CAD build for the part. Positions are in the model's coordinates, mm. Coordinates: 2 decimals unless noted, no trailing zeros. Answer in a Markdown table with one row per item. Add a question column.
Q1. Drill centre lines: line 1 along Y through (x, z) = (-9, 0.65); line 2 along X through (y, z) = (104.2, 0.55); line 3 along Y through (x, z) = (0, 0.75). Where is each one in solid material? Low to high. Write a range as from..to.
Q2. Band-saw the part on A-A (z = 1.3). State how many separate pieces and enclosed holes the cut face has, and give its area (3 significant figures).
Q3. Pin check, flat tip, straight feed: pin 1 (6 mm diameter, centred on x = -19, y = -42, fed in from -Z). Stop position of the tip, or through.
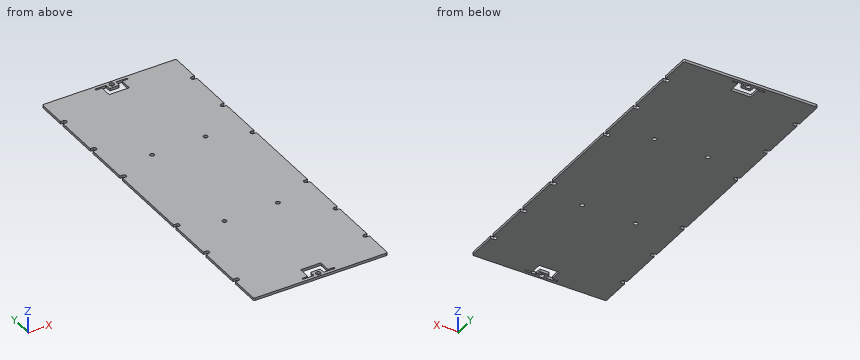
```python
from build123d import *

# Parameters (mm, degrees)
SKETCH1_W                  = 82.8
SKETCH1_H                  = 213.8
SKETCH1_R                  = 0.8
PCB_EXTRUDE_DEPTH          = 1.6
SKETCH7_W                  = 82.5
SKETCH7_H                  = 213.5
OFFSET_EDGES_DEPTH         = 1.6
CORNER_FILLETS_ON_PCB_R    = 1
SKETCH3_R                  = 1.5
SOLAR_HOLE_DEPTH           = 1.6
FILLETS_FOR_SOLAR_HOLE_R   = 0.5
M2_CLEARANCE_HOLE1_D       = 2.6
SKETCH6_W                  = 1.75
SKETCH6_H                  = 2.6
SLOTS_FOR_EDGE_HOLES_DEPTH = 1.6


with BuildPart() as part:
    # Sketch1 → pcb extrude (new body)
    with BuildSketch(Plane.XY):
        Rectangle(SKETCH1_W, SKETCH1_H)
        with Locations((-39.5, -27)):
            Circle(SKETCH1_R, mode=Mode.SUBTRACT)
        with Locations((39.5, -27)):
            Circle(SKETCH1_R, mode=Mode.SUBTRACT)
        with Locations((-39.5, 87)):
            Circle(SKETCH1_R, mode=Mode.SUBTRACT)
        with Locations((-39.5, 57)):
            Circle(SKETCH1_R, mode=Mode.SUBTRACT)
        with Locations((-39.5, 27)):
            Circle(SKETCH1_R, mode=Mode.SUBTRACT)
        with Locations((-16.5, 36.5)):
            Circle(SKETCH1_R, mode=Mode.SUBTRACT)
        with Locations((-16.5, -36.5)):
            Circle(SKETCH1_R, mode=Mode.SUBTRACT)
        with Locations((-39.5, -57)):
            Circle(SKETCH1_R, mode=Mode.SUBTRACT)
        with Locations((-39.5, -87)):
            Circle(SKETCH1_R, mode=Mode.SUBTRACT)
        with Locations((0, -104.2)):
            Circle(SKETCH1_R, mode=Mode.SUBTRACT)
        with Locations((39.5, -87)):
            Circle(SKETCH1_R, mode=Mode.SUBTRACT)
        with Locations((39.5, -57)):
            Circle(SKETCH1_R, mode=Mode.SUBTRACT)
        with Locations((16.5, -36.5)):
            Circle(SKETCH1_R, mode=Mode.SUBTRACT)
        with Locations((39.5, 27)):
            Circle(SKETCH1_R, mode=Mode.SUBTRACT)
        with Locations((16.5, 36.5)):
            Circle(SKETCH1_R, mode=Mode.SUBTRACT)
        with Locations((39.5, 57)):
            Circle(SKETCH1_R, mode=Mode.SUBTRACT)
        with Locations((39.5, 87)):
            Circle(SKETCH1_R, mode=Mode.SUBTRACT)
        with Locations((0, 104.2)):
            Circle(SKETCH1_R, mode=Mode.SUBTRACT)
    extrude(amount=PCB_EXTRUDE_DEPTH)

    # Sketch7 → Offset Edges (cut)
    with BuildSketch(Plane.XY.offset(1.6)):
        Polygon((-41.25, 106.9), (-41.4, 106.9), (-41.4, -106.9), (-41.25, -106.9), (41.25, -106.9), (41.4, -106.9), (41.4, 106.9), (41.25, 106.9), align=None)
        Rectangle(SKETCH7_W, SKETCH7_H, mode=Mode.SUBTRACT)
    extrude(amount=-OFFSET_EDGES_DEPTH, mode=Mode.SUBTRACT)

    # corner fillets on PCB
    corner_fillets_on_pcb_edges = [part.edges().sort_by_distance(p)[0] for p in [
        (41.25, -106.75, 0.8),
        (41.25, 106.75, 0.8),
        (-41.25, 106.75, 0.8),
        (-41.25, -106.75, 0.8),
    ]]
    fillet(corner_fillets_on_pcb_edges, radius=CORNER_FILLETS_ON_PCB_R)

    # Sketch3 → Solar Hole (cut)
    with BuildSketch(Plane.XY.offset(1.6)):
        with Locations((0, 104.2)):
            Circle(SKETCH3_R)
        with BuildLine():
            Line((-3, 101.4), (3, 101.4))
            Line((3, 101.4), (3, 104.9))
            Line((3, 104.9), (9.5, 104.9))
            ThreePointArc((9.5, 104.9), (10, 104.4), (9.5, 103.9))
            Line((9.5, 103.9), (6.2, 103.9))
            Line((6.2, 103.9), (6.2, 96.6))
            Line((6.2, 96.6), (-6.2, 96.6))
            Line((-6.2, 96.6), (-6.2, 103.9))
            Line((-6.2, 103.9), (-9.5, 103.9))
            ThreePointArc((-9.5, 103.9), (-10, 104.4), (-9.5, 104.9))
            Line((-9.5, 104.9), (-3, 104.9))
            Line((-3, 104.9), (-3, 101.4))
        make_face()
    solar_hole = extrude(amount=-SOLAR_HOLE_DEPTH, mode=Mode.SUBTRACT)

    # Mirror solar hole: Solar Hole across plane
    add(solar_hole.mirror(Plane.ZX), mode=Mode.SUBTRACT)

    # fillets for solar hole
    fillets_for_solar_hole_edges = [part.edges().sort_by_distance(p)[0] for p in [
        (6.2, 103.9, 0.8),
        (6.2, 96.6, 0.8),
        (-6.2, 96.6, 0.8),
        (-6.2, 103.9, 0.8),
        (-3, 104.9, 0.8),
        (-3, 101.4, 0.8),
        (3, 101.4, 0.8),
        (3, 104.9, 0.8),
        (6.2, -103.9, 0.8),
        (6.2, -96.6, 0.8),
        (-6.2, -96.6, 0.8),
        (-6.2, -103.9, 0.8),
        (-3, -104.9, 0.8),
        (-3, -101.4, 0.8),
        (3, -101.4, 0.8),
        (3, -104.9, 0.8),
    ]]
    fillet(fillets_for_solar_hole_edges, radius=FILLETS_FOR_SOLAR_HOLE_R)

    # M2 Clearance Hole1 (through all)
    with Locations(Plane(origin=(0, 0, 0), x_dir=(-1, 0, 0), z_dir=(0, 0, -1))):
        with Locations((39.5, 87), (-39.5, 87), (16.5, 36.5), (-16.5, 36.5), (39.5, 57), (-39.5, 57), (39.5, 27), (-39.5, 27), (39.5, -57), (16.5, -36.5), (-16.5, -36.5), (-39.5, -57), (-39.5, -87), (39.5, -87), (39.5, -27), (-39.5, -27)):
            Hole(M2_CLEARANCE_HOLE1_D / 2)

    # Sketch6 → slots for edge holes (cut)
    with BuildSketch(Plane.XY.offset(1.6)):
        with Locations((-40.375, 87)):
            Rectangle(SKETCH6_W, SKETCH6_H)
        with Locations((40.375, 87)):
            Rectangle(SKETCH6_W, SKETCH6_H)
        with Locations((40.375, 57)):
            Rectangle(SKETCH6_W, SKETCH6_H)
        with Locations((40.375, 27)):
            Rectangle(SKETCH6_W, SKETCH6_H)
        with Locations((-40.375, 57)):
            Rectangle(SKETCH6_W, SKETCH6_H)
        with Locations((-40.375, 27)):
            Rectangle(SKETCH6_W, SKETCH6_H)
        with Locations((40.375, -87)):
            Rectangle(SKETCH6_W, SKETCH6_H)
        with Locations((-40.375, -87)):
            Rectangle(SKETCH6_W, SKETCH6_H)
        with Locations((40.375, -57)):
            Rectangle(SKETCH6_W, SKETCH6_H)
        with Locations((40.375, -27)):
            Rectangle(SKETCH6_W, SKETCH6_H)
        with Locations((-40.375, -57)):
            Rectangle(SKETCH6_W, SKETCH6_H)
        with Locations((-40.375, -27)):
            Rectangle(SKETCH6_W, SKETCH6_H)
    extrude(amount=-SLOTS_FOR_EDGE_HOLES_DEPTH, mode=Mode.SUBTRACT)


solid = part.part
```
Checked values:
| question | item | result |
|---|---|---|
| 1 | line 1 | y = -106.75..-104.9, -103.9..103.9, 104.9..106.75 |
| 1 | line 2 | x = -41.25..-9.96, -3..-1.5, 1.5..3, 9.96..41.25 |
| 1 | line 3 | y = -106.75..-105.7, -102.7..-101.4, -96.6..96.6, 101.4..102.7, 105.7..106.75 |
| 2 | separate pieces | 1 |
| 2 | enclosed holes | 8 |
| 2 | area | 17,300 mm² |
| 3 | pin 1 | stops at z = 0 |
